The listing builds one solid part. Answer for the finished solid, in the listing's coordinates (mm). Round coordinates to 2 decimals unless told otherwise and drop trailing zeros. Write each loop counter-clockwise with the first axis right and the second up, starting at its lowest first coordinate (ties: lowest second). Pieces come first, ordered by that corner, then holes.
(1) Each of these flat-tipped pins is pushed along its axis until it touches: pin 1 Ø3 at (y, z) = (21, 4.5) entering from -X; pin 2 Ø0.8 at (y, z) = (2.5, 6.5) entering from +X; pin 3 Ø1.5 at (x, z) = (7.5, 1) entering from +Y. Where does it stop, or does it pass through?
(2) A cutting plane is placed at A-A, the plane z = 2. Give the vertices of the cut face in (x, y) (3 decimals).
(3) Find the intervals of material crossed by probe 1 along X at (y, z) = (-2.5, 6.25); probe 2 along Z at (x, y) = (1.5, -10.5); probe 3 along Z at (x, y) = (23, -14.5), in increasing order.
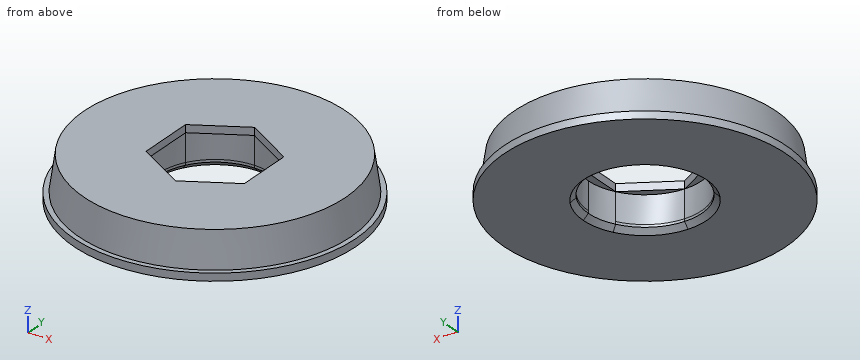
from build123d import *

# Parameters (mm, degrees)
F5_R          = 27
F6_DEPTH      = 7
F5_R_2        = 28
F7_DEPTH      = 1.5
F8_DEPTH      = 7.001
F8_DEPTH_BACK = 1.501
F9_DEPTH      = 5.5
F9_DEPTH_BACK = 1.501
F10_SIZE2     = 0.99999
F10_SIZE      = 6.99999
F11_SIZE      = 1


# Not quite as in the source:
# - a fillet or chamfer is up to 0.001 mm smaller than in the source, because OpenCascade refuses the exact size


with BuildPart() as f6:
    # F5 (on Top) → F6 (new body)
    with BuildSketch(Plane.XY):
        Circle(F5_R)
        with BuildLine():
            ThreePointArc((9.7427857926, 5.625), (10.8666655458, 2.9117142574), (11.25, 0))
            ThreePointArc((11.25, 0), (10.8666655458, -2.9117142574), (9.7427857926, -5.625))
            ThreePointArc((9.7427857926, -5.625), (5.625, -9.7427857926), (0, -11.25))
            ThreePointArc((0, -11.25), (-5.625, -9.7427857926), (-9.7427857926, -5.625))
            ThreePointArc((-9.7427857926, -5.625), (-11.25, 0), (-9.7427857926, 5.625))
            ThreePointArc((-9.7427857926, 5.625), (-5.625, 9.7427857926), (0, 11.25))
            ThreePointArc((0, 11.25), (5.625, 9.7427857926), (9.7427857926, 5.625))
        make_face(mode=Mode.SUBTRACT)
        with BuildLine():
            Line((-9.7427857926, -5.625), (-9.7427857926, 5.625))
            ThreePointArc((-9.7427857926, 5.625), (-11.25, 0), (-9.7427857926, -5.625))
        make_face()
        with BuildLine():
            Line((0, 11.25), (9.7427857926, 5.625))
            ThreePointArc((9.7427857926, 5.625), (5.625, 9.7427857926), (0, 11.25))
        make_face()
        with BuildLine():
            ThreePointArc((9.7427857926, -5.625), (10.8666655458, -2.9117142574), (11.25, 0))
            ThreePointArc((11.25, 0), (10.8666655458, 2.9117142574), (9.7427857926, 5.625))
            Line((9.7427857926, 5.625), (9.7427857926, -5.625))
        make_face()
        with BuildLine():
            ThreePointArc((0, -11.25), (5.625, -9.7427857926), (9.7427857926, -5.625))
            Line((9.7427857926, -5.625), (0, -11.25))
        make_face()
        with BuildLine():
            ThreePointArc((-9.7427857926, -5.625), (-5.625, -9.7427857926), (0, -11.25))
            Line((0, -11.25), (-9.7427857926, -5.625))
        make_face()
        with BuildLine():
            Line((-9.7427857926, 5.625), (0, 11.25))
            ThreePointArc((0, 11.25), (-5.625, 9.7427857926), (-9.7427857926, 5.625))
        make_face()
        Polygon((9.7427857926, -5.625), (9.7427857926, 5.625), (0, 11.25), (-9.7427857926, 5.625), (-9.7427857926, -5.625), (0, -11.25), align=None)
    extrude(amount=F6_DEPTH)

    # F5 (on Top) → F7 (join)
    with BuildSketch(Plane.XY):
        Circle(F5_R_2)
        Circle(F5_R, mode=Mode.SUBTRACT)
        Circle(F5_R)
        with BuildLine():
            ThreePointArc((9.7427857926, 5.625), (10.8666655458, 2.9117142574), (11.25, 0))
            ThreePointArc((11.25, 0), (10.8666655458, -2.9117142574), (9.7427857926, -5.625))
            ThreePointArc((9.7427857926, -5.625), (5.625, -9.7427857926), (0, -11.25))
            ThreePointArc((0, -11.25), (-5.625, -9.7427857926), (-9.7427857926, -5.625))
            ThreePointArc((-9.7427857926, -5.625), (-11.25, 0), (-9.7427857926, 5.625))
            ThreePointArc((-9.7427857926, 5.625), (-5.625, 9.7427857926), (0, 11.25))
            ThreePointArc((0, 11.25), (5.625, 9.7427857926), (9.7427857926, 5.625))
        make_face(mode=Mode.SUBTRACT)
        Polygon((9.7427857926, -5.625), (9.7427857926, 5.625), (0, 11.25), (-9.7427857926, 5.625), (-9.7427857926, -5.625), (0, -11.25), align=None)
        with BuildLine():
            ThreePointArc((9.7427857926, -5.625), (10.8666655458, -2.9117142574), (11.25, 0))
            ThreePointArc((11.25, 0), (10.8666655458, 2.9117142574), (9.7427857926, 5.625))
            Line((9.7427857926, 5.625), (9.7427857926, -5.625))
        make_face()
        with BuildLine():
            ThreePointArc((0, -11.25), (5.625, -9.7427857926), (9.7427857926, -5.625))
            Line((9.7427857926, -5.625), (0, -11.25))
        make_face()
        with BuildLine():
            ThreePointArc((-9.7427857926, -5.625), (-5.625, -9.7427857926), (0, -11.25))
            Line((0, -11.25), (-9.7427857926, -5.625))
        make_face()
        with BuildLine():
            Line((-9.7427857926, -5.625), (-9.7427857926, 5.625))
            ThreePointArc((-9.7427857926, 5.625), (-11.25, 0), (-9.7427857926, -5.625))
        make_face()
        with BuildLine():
            Line((0, 11.25), (9.7427857926, 5.625))
            ThreePointArc((9.7427857926, 5.625), (5.625, 9.7427857926), (0, 11.25))
        make_face()
        with BuildLine():
            Line((-9.7427857926, 5.625), (0, 11.25))
            ThreePointArc((0, 11.25), (-5.625, 9.7427857926), (-9.7427857926, 5.625))
        make_face()
    extrude(amount=-F7_DEPTH)

    # F5 (on Top) → F8 (cut, two sides)
    with BuildSketch(Plane.XY) as f8_sk:
        Polygon((9.7427857926, -5.625), (9.7427857926, 5.625), (0, 11.25), (-9.7427857926, 5.625), (-9.7427857926, -5.625), (0, -11.25), align=None)
    extrude(amount=F8_DEPTH, mode=Mode.SUBTRACT)
    extrude(f8_sk.sketch, amount=-F8_DEPTH_BACK, mode=Mode.SUBTRACT)

    # F5 (on Top) → F9 (cut, two sides)
    with BuildSketch(Plane.XY) as f9_sk:
        with BuildLine():
            ThreePointArc((-9.7427857926, -5.625), (-5.625, -9.7427857926), (0, -11.25))
            Line((0, -11.25), (-9.7427857926, -5.625))
        make_face()
        with BuildLine():
            ThreePointArc((0, -11.25), (5.625, -9.7427857926), (9.7427857926, -5.625))
            Line((9.7427857926, -5.625), (0, -11.25))
        make_face()
        with BuildLine():
            ThreePointArc((9.7427857926, -5.625), (10.8666655458, -2.9117142574), (11.25, 0))
            ThreePointArc((11.25, 0), (10.8666655458, 2.9117142574), (9.7427857926, 5.625))
            Line((9.7427857926, 5.625), (9.7427857926, -5.625))
        make_face()
        with BuildLine():
            Line((0, 11.25), (9.7427857926, 5.625))
            ThreePointArc((9.7427857926, 5.625), (5.625, 9.7427857926), (0, 11.25))
        make_face()
        with BuildLine():
            Line((-9.7427857926, 5.625), (0, 11.25))
            ThreePointArc((0, 11.25), (-5.625, 9.7427857926), (-9.7427857926, 5.625))
        make_face()
        with BuildLine():
            Line((-9.7427857926, -5.625), (-9.7427857926, 5.625))
            ThreePointArc((-9.7427857926, 5.625), (-11.25, 0), (-9.7427857926, -5.625))
        make_face()
    extrude(amount=F9_DEPTH, mode=Mode.SUBTRACT)
    extrude(f9_sk.sketch, amount=-F9_DEPTH_BACK, mode=Mode.SUBTRACT)

    # F10 (size 7 and 1 in the source; OpenCascade refuses exactly that, so slightly less here)
    f10_edges = [f6.edges().sort_by_distance(p)[0] for p in [
        (-27, 0, 7),
    ]]
    f10_side = f6.faces().sort_by_distance((-27, 0, 3.5))[0]
    chamfer(f10_edges, length=F10_SIZE, length2=F10_SIZE2, reference=f10_side)

    # F11
    f11_edges = [f6.edges().sort_by_distance(p)[0] for p in [
        (0, 11.25, -1.5),
    ]]
    chamfer(f11_edges, length=F11_SIZE)


solid = f6.part
Solutions:
1. pin 1: stops at x = -17.76
1. pin 2: stops at x = 26.02
1. pin 3: stops at y = 26.02
2. outline: circle Ø53.429 at (0, 0); hole circle Ø22.5 at (0, 0)
3. probe 1: x = -25.99 to -9.74, 9.74 to 25.99
3. probe 2: z = 5.5 to 7
3. probe 3: z = -1.5 to 0
